Work out the finished part from the listing and answer in its coordinate system (mm). Face numbers are marked on the shaded views. A direction names the side the tool comes from. Give positions to 0.01 mm unless a question says otherwise; leave off trailing zeros. Loops run counter-clockwise (first coordinate to the right, second up) from the corner with the lowest first, then second, coordinate; pieces in that order, holes last.
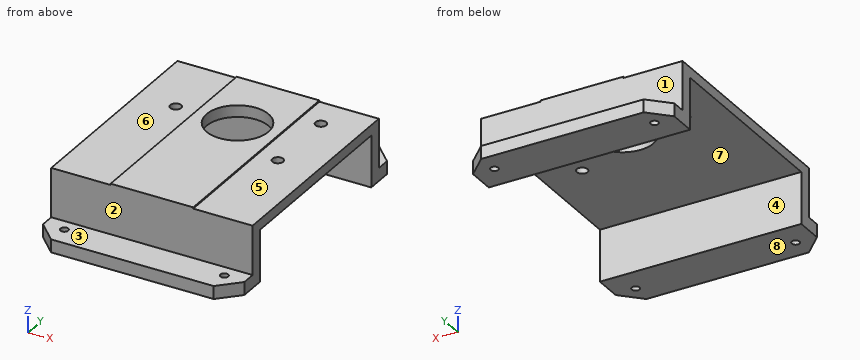
```python
from build123d import *

# Parameters (mm, degrees)
EXTRUDE_1_DEPTH     = 5
EXTRUDE_1_2_DEPTH   = 5
EXTRUDE_2_DEPTH     = 78
CUT_EXTRUDE_1_REACH = 73.568
SKETCH_4_R          = 12
EXTRUDE_START       = 0.5
SKETCH_5_W          = 32
SKETCH_5_H          = 84
SKETCH_5_R          = 12
EXTRUDE_3_DEPTH     = 0.5
CUT_EXTRUDE_2_REACH = 73.568
SKETCH_6_R          = 2.1
CUT_EXTRUDE_3_REACH = 72.187
SKETCH_7_R          = 1.5


with BuildPart() as part:
    # Sketch 2 → Extrude 1 (new body)
    with BuildSketch(Plane.XY):
        Polygon((39, 42), (-39, 42), (-39, 47.485281374), (-31.485281374, 55), (31.485281374, 55), (39, 47.485281374), align=None)
    extrude(amount=EXTRUDE_1_DEPTH)



with BuildPart() as body_2:
    # Sketch 2 → Extrude 1 2 (new body)
    with BuildSketch(Plane.XY):
        Polygon((31.485281374, -55), (-31.485281374, -55), (-39, -47.485281374), (-39, -42), (39, -42), (39, -47.485281374), align=None)
    extrude(amount=EXTRUDE_1_2_DEPTH)


with BuildPart() as part_1:
    add(part.part)

    add(body_2.part)  # Extrude 2 merges body 2
    # Sketch 3 → Extrude 2 (add)
    with BuildSketch(Plane.ZY.offset(39)):
        Polygon((0, 42), (24, 42), (24, -42), (0, -42), (0, -37), (20, -37), (20, 37), (0, 37), align=None)
    extrude(amount=-EXTRUDE_2_DEPTH)

    # Sketch 4 → Cut-Extrude 1 (cut, up to next)
    with BuildSketch(Plane.XY.offset(24), mode=Mode.PRIVATE) as cut_extrude_1_sk1:
        with Locations((0, 15)):
            Circle(SKETCH_4_R)
    cut_extrude_1_tool1 = extrude(cut_extrude_1_sk1.sketch, amount=-CUT_EXTRUDE_1_REACH, mode=Mode.PRIVATE) & part_1.part
    add(cut_extrude_1_tool1.solids().sort_by_distance((0, 15, 24))[0], mode=Mode.SUBTRACT)

    # Sketch 5 → Extrude 3 (add)
    with BuildSketch(Plane.XY.offset(24).offset(EXTRUDE_START)):
        Rectangle(SKETCH_5_W, SKETCH_5_H)
        with Locations((0, 15)):
            Circle(SKETCH_5_R, mode=Mode.SUBTRACT)
    extrude(amount=-EXTRUDE_3_DEPTH)

    # Sketch 6 → Cut-Extrude 2 (cut, up to next)
    with BuildSketch(Plane.XY.offset(24), mode=Mode.PRIVATE) as cut_extrude_2_sk1:
        with Locations((-23.95, 15)):
            Circle(SKETCH_6_R)
    cut_extrude_2_tool1 = extrude(cut_extrude_2_sk1.sketch, amount=-CUT_EXTRUDE_2_REACH, mode=Mode.PRIVATE) & part_1.part
    # Sketch 6 → Cut-Extrude 2 (cut, up to next)
    with BuildSketch(Plane.XY.offset(24), mode=Mode.PRIVATE) as cut_extrude_2_sk2:
        with Locations((23.95, 29.35)):
            Circle(SKETCH_6_R)
    cut_extrude_2_tool2 = extrude(cut_extrude_2_sk2.sketch, amount=-CUT_EXTRUDE_2_REACH, mode=Mode.PRIVATE) & part_1.part
    # Sketch 6 → Cut-Extrude 2 (cut, up to next)
    with BuildSketch(Plane.XY.offset(24), mode=Mode.PRIVATE) as cut_extrude_2_sk3:
        with Locations((23.95, 0.65)):
            Circle(SKETCH_6_R)
    cut_extrude_2_tool3 = extrude(cut_extrude_2_sk3.sketch, amount=-CUT_EXTRUDE_2_REACH, mode=Mode.PRIVATE) & part_1.part
    add(cut_extrude_2_tool1.solids().sort_by_distance((-23.95, 15, 24))[0], mode=Mode.SUBTRACT)
    add(cut_extrude_2_tool2.solids().sort_by_distance((23.95, 29.35, 24))[0], mode=Mode.SUBTRACT)
    add(cut_extrude_2_tool3.solids().sort_by_distance((23.95, 0.65, 24))[0], mode=Mode.SUBTRACT)

    # Sketch 7 → Cut-Extrude 3 (cut, up to next)
    with BuildSketch(Plane.XY.offset(5), mode=Mode.PRIVATE) as cut_extrude_3_sk1:
        with Locations((-31, 47)):
            Circle(SKETCH_7_R)
    cut_extrude_3_tool1 = extrude(cut_extrude_3_sk1.sketch, amount=-CUT_EXTRUDE_3_REACH, mode=Mode.PRIVATE) & part_1.part
    # Sketch 7 → Cut-Extrude 3 (cut, up to next)
    with BuildSketch(Plane.XY.offset(5), mode=Mode.PRIVATE) as cut_extrude_3_sk2:
        with Locations((31, 47)):
            Circle(SKETCH_7_R)
    cut_extrude_3_tool2 = extrude(cut_extrude_3_sk2.sketch, amount=-CUT_EXTRUDE_3_REACH, mode=Mode.PRIVATE) & part_1.part
    # Sketch 7 → Cut-Extrude 3 (cut, up to next)
    with BuildSketch(Plane.XY.offset(5), mode=Mode.PRIVATE) as cut_extrude_3_sk3:
        with Locations((31, -47)):
            Circle(SKETCH_7_R)
    cut_extrude_3_tool3 = extrude(cut_extrude_3_sk3.sketch, amount=-CUT_EXTRUDE_3_REACH, mode=Mode.PRIVATE) & part_1.part
    # Sketch 7 → Cut-Extrude 3 (cut, up to next)
    with BuildSketch(Plane.XY.offset(5), mode=Mode.PRIVATE) as cut_extrude_3_sk4:
        with Locations((-31, -47)):
            Circle(SKETCH_7_R)
    cut_extrude_3_tool4 = extrude(cut_extrude_3_sk4.sketch, amount=-CUT_EXTRUDE_3_REACH, mode=Mode.PRIVATE) & part_1.part
    add(cut_extrude_3_tool1.solids().sort_by_distance((-31, 47, 5))[0], mode=Mode.SUBTRACT)
    add(cut_extrude_3_tool2.solids().sort_by_distance((31, 47, 5))[0], mode=Mode.SUBTRACT)
    add(cut_extrude_3_tool3.solids().sort_by_distance((31, -47, 5))[0], mode=Mode.SUBTRACT)
    add(cut_extrude_3_tool4.solids().sort_by_distance((-31, -47, 5))[0], mode=Mode.SUBTRACT)


solid = part_1.part
```
Q1. Determine the mould class of the marked faces 1, 2, 3 and 4 for opening direction Y: +Y half, -Y half, draft (parallel to the pull), parting line (faces both ways), or undercut.
Q2. Section A-A on y = 29.35 is taken. Give the vertices of the cut face in (x, z), plus the area to 3 significant figures.
Q3. Section D-D on x = -23.95 is taken. Give the vertices of the cut face in (y, z).
Q4. Given pin 1 (5 mm diameter, centred on x = 23.95, y = 29.35, fed in from -Z); pin 2 (5 mm diameter, centred on x = -6, z = 8, fed in from -Y); pin 3 (3 mm diameter, centred on x = -16.5, z = 21, fed in from +Y), each flat-ended and moving along its own axis, determine where each tip first touches the part or whether it passes through.
Q5. Consider line 1 along Y through (x, z) = (31, 3.85); line 2 along Y through (x, z) = (-16, 3.5); line 3 along Z through (x, y) = (30, 30). Determine where each line is inside the solid, lowest interval first.
Q6. Section C-C on z = 10.25 is taken. Give the vertices of the cut face in (x, y).
Q7. Section B-B on x = 23.95 is taken. Give the vertices of the cut face in (y, z), plus the area to 3 significant figures.
Q8. Which of the six approach directions +Z, -Z, +X, -X, +Y, -Y give full straight-line access (tool end or side, diameter ignored) to the marked faces 5, 6, 7 and 8?
Check result:
1. face 1: +Y half
1. face 2: -Y half
1. face 3: draft
1. face 4: undercut
2. outline: (-39, 20) - (21.85, 20) - (21.85, 24) - (16, 24) - (16, 24.5) - (-16, 24.5) - (-16, 24) - (-39, 24) - close; (26.05, 20) - (39, 20) - (39, 24) - (26.05, 24) - close
2. area: 311 mm2
3. outline: (-55, 0) - (-37, 0) - (-37, 20) - (12.9, 20) - (12.9, 24) - (-42, 24) - (-42, 5) - (-55, 5) - close; (17.1, 20) - (37, 20) - (37, 0) - (55, 0) - (55, 5) - (42, 5) - (42, 24) - (17.1, 24) - close
4. pin 1: stops at z = 20
4. pin 2: stops at y = -42
4. pin 3: stops at y = 42
5. line 1: y = -55 to -48.5, -45.5 to -37, 37 to 45.5, 48.5 to 55
5. line 2: y = -55 to -37, 37 to 55
5. line 3: z = 20 to 24
6. outline: (-39, -42) - (39, -42) - (39, -37) - (-39, -37) - close; (-39, 37) - (39, 37) - (39, 42) - (-39, 42) - close
7. outline: (-55, 0) - (-37, 0) - (-37, 20) - (-1.45, 20) - (-1.45, 24) - (-42, 24) - (-42, 5) - (-55, 5) - close; (2.75, 20) - (27.25, 20) - (27.25, 24) - (2.75, 24) - close; (31.45, 20) - (37, 20) - (37, 0) - (55, 0) - (55, 5) - (42, 5) - (42, 24) - (31.45, 24) - close
7. area: 632 mm2
8. face 5: +Z, +X, +Y, -Y
8. face 6: +Z, -X, +Y, -Y
8. face 7: -Z, +X, -X
8. face 8: -Z, +X, -X, +Y, -Y
